Read the model definition and answer for the solid it produces. Units are mm, in the model's axes. A direction names the side the tool comes from. Give positions to 0.01 mm unless a question says otherwise; leave off trailing zeros. Write each loop counter-clockwise with the first axis right and the second up, starting at its lowest first coordinate (ties: lowest second). Pieces come first, ordered by that corner, then holes. Notation, with made-up numbers: M -23,35 L 12,35 A21 ccw 12,65 Z; hole C 2,28.25 d11. An arc over 180 degrees is marked long. Put each result on its own line as item: value.
from build123d import *

# Parameters (mm, degrees)
ESBO_O1_R                                            = 7
RESSALTO_EXTRUS_O1_DEPTH                             = 7.9375
ESCAREADO_PARA_PARAFUSO_DE_M_QUINA_COM_C_D           = 5.5
ESCAREADO_PARA_PARAFUSO_DE_M_QUINA_COM_C_DEPTH       = 30
ESCAREADO_PARA_PARAFUSO_DE_M_QUINA_COM_C_CSINK_D     = 10.4
ESCAREADO_PARA_PARAFUSO_DE_M_QUINA_COM_C_CSINK_ANGLE = 90
ESCAREADO_PARA_PARAFUSO_DE_M_QUINA_COM_C_TIP         = 1.652366702
ESCAREADO_PARA_PARAFUSO_DE_M_QUINA_C_2_D             = 6.6
ESCAREADO_PARA_PARAFUSO_DE_M_QUINA_C_2_DEPTH         = 30
ESCAREADO_PARA_PARAFUSO_DE_M_QUINA_C_2_CSINK_D       = 12.6
ESCAREADO_PARA_PARAFUSO_DE_M_QUINA_C_2_CSINK_ANGLE   = 90
ESCAREADO_PARA_PARAFUSO_DE_M_QUINA_C_2_TIP           = 1.982840043
BROCA_DE_ROSQUEAR_PARA_TARRAXA_DE_M5X0_8_D           = 4.2
BROCA_DE_ROSQUEAR_PARA_TARRAXA_DE_M5X0_8_DEPTH       = 20
BROCA_DE_ROSQUEAR_PARA_TARRAXA_DE_M5X0_8_TIP         = 1.2618073
BROCA_DE_ROSQUEAR_PARA_TARRAXA_DE_M5_2_D             = 4.2
BROCA_DE_ROSQUEAR_PARA_TARRAXA_DE_M5_2_DEPTH         = 20
BROCA_DE_ROSQUEAR_PARA_TARRAXA_DE_M5_2_TIP           = 1.2618073
BROCA_DE_ROSQUEAR_PARA_TARRAXA_DE_M6X1_0_D           = 5
BROCA_DE_ROSQUEAR_PARA_TARRAXA_DE_M6X1_0_DEPTH       = 15
BROCA_DE_ROSQUEAR_PARA_TARRAXA_DE_M6X1_0_TIP         = 1.502151548
FILLET1_R                                            = 6
SKETCH7_R                                            = 9.5
CUT_EXTRUDE4_DEPTH                                   = 5


with BuildPart() as part:
    # Esboço1 → Ressalto-extrusão1 (new, symmetric)
    with BuildSketch(Plane(origin=(0, 0, 0), x_dir=(0, 0, -1), z_dir=(1, 0, 0))):
        Polygon((-10, 38.5), (-40, 38.5), (-40, 23.5), (-40, 17.44427191), (-32, 8.5), (-32, -16.5), (73, -16.5), (73, 27.5), (-10, 27.5), align=None)
        with Locations((-25, 23.5)):
            Circle(ESBO_O1_R, mode=Mode.SUBTRACT)
    extrude(amount=RESSALTO_EXTRUS_O1_DEPTH, both=True)

    # Escareado para parafuso de m_quina com c
    with Locations(Plane(origin=(33.0625, -10.251665499, 40.070399895), x_dir=(1, 0, 0), z_dir=(0, 0, 1))):
        with Locations((-33.0625, 13.751665499), (-33.0625, -1.248334501), (33.0625, -1.248334501), (33.0625, 13.751665499)):
            CounterSinkHole(ESCAREADO_PARA_PARAFUSO_DE_M_QUINA_COM_C_D / 2, ESCAREADO_PARA_PARAFUSO_DE_M_QUINA_COM_C_CSINK_D / 2, depth=ESCAREADO_PARA_PARAFUSO_DE_M_QUINA_COM_C_DEPTH, counter_sink_angle=ESCAREADO_PARA_PARAFUSO_DE_M_QUINA_COM_C_CSINK_ANGLE)
            with Locations((0, 0, -(ESCAREADO_PARA_PARAFUSO_DE_M_QUINA_COM_C_DEPTH + ESCAREADO_PARA_PARAFUSO_DE_M_QUINA_COM_C_TIP / 2))):  # 118° drill point
                Cone(0, ESCAREADO_PARA_PARAFUSO_DE_M_QUINA_COM_C_D / 2, ESCAREADO_PARA_PARAFUSO_DE_M_QUINA_COM_C_TIP, mode=Mode.SUBTRACT)

    # Escareado para parafuso de m_quina c 2
    with Locations(Plane(origin=(33.0625, -23.5, -11.460196829), x_dir=(-1, 0, 0), z_dir=(0, -1, 0))):
        with Locations((33.06, 53.539803171), (33.06, -3.413475694), (-33.06, -3.413475694), (-33.06, 49.586524306)):
            CounterSinkHole(ESCAREADO_PARA_PARAFUSO_DE_M_QUINA_C_2_D / 2, ESCAREADO_PARA_PARAFUSO_DE_M_QUINA_C_2_CSINK_D / 2, depth=ESCAREADO_PARA_PARAFUSO_DE_M_QUINA_C_2_DEPTH, counter_sink_angle=ESCAREADO_PARA_PARAFUSO_DE_M_QUINA_C_2_CSINK_ANGLE)
            with Locations((0, 0, -(ESCAREADO_PARA_PARAFUSO_DE_M_QUINA_C_2_DEPTH + ESCAREADO_PARA_PARAFUSO_DE_M_QUINA_C_2_TIP / 2))):  # 118° drill point
                Cone(0, ESCAREADO_PARA_PARAFUSO_DE_M_QUINA_C_2_D / 2, ESCAREADO_PARA_PARAFUSO_DE_M_QUINA_C_2_TIP, mode=Mode.SUBTRACT)

    # Broca de rosquear para tarraxa de M5x0.8
    with Locations(Plane(origin=(33.0625, 48.5, -11.460196829), x_dir=(1, 0, 0), z_dir=(0, 1, 0))):
        with Locations((33.06, -45.460196829), (-33.065, -45.460196829)):
            Hole(BROCA_DE_ROSQUEAR_PARA_TARRAXA_DE_M5X0_8_D / 2, depth=BROCA_DE_ROSQUEAR_PARA_TARRAXA_DE_M5X0_8_DEPTH)
            with Locations((0, 0, -(BROCA_DE_ROSQUEAR_PARA_TARRAXA_DE_M5X0_8_DEPTH + BROCA_DE_ROSQUEAR_PARA_TARRAXA_DE_M5X0_8_TIP / 2))):  # 118° drill point
                Cone(0, BROCA_DE_ROSQUEAR_PARA_TARRAXA_DE_M5X0_8_D / 2, BROCA_DE_ROSQUEAR_PARA_TARRAXA_DE_M5X0_8_TIP, mode=Mode.SUBTRACT)

    # Broca de rosquear para tarraxa de M5 2
    with Locations(Plane(origin=(33.0625, -10.251665499, 0), x_dir=(-1, 0, 0), z_dir=(0, 0, -1))):
        with Locations((-33.06, 43.751665499), (33.065, 43.751665499)):
            Hole(BROCA_DE_ROSQUEAR_PARA_TARRAXA_DE_M5_2_D / 2, depth=BROCA_DE_ROSQUEAR_PARA_TARRAXA_DE_M5_2_DEPTH)
            with Locations((0, 0, -(BROCA_DE_ROSQUEAR_PARA_TARRAXA_DE_M5_2_DEPTH + BROCA_DE_ROSQUEAR_PARA_TARRAXA_DE_M5_2_TIP / 2))):  # 118° drill point
                Cone(0, BROCA_DE_ROSQUEAR_PARA_TARRAXA_DE_M5_2_D / 2, BROCA_DE_ROSQUEAR_PARA_TARRAXA_DE_M5_2_TIP, mode=Mode.SUBTRACT)

    # Broca de rosquear para tarraxa de M6x1.01
    with Locations(Plane(origin=(33.0625, 27.5, -11.460196829), x_dir=(1, 0, 0), z_dir=(0, 1, 0))):
        with Locations((33.06, 49.539803171), (-33.06, 53.539803171), (-33.06, -3.413475694), (33.06, -3.413475694)):
            Hole(BROCA_DE_ROSQUEAR_PARA_TARRAXA_DE_M6X1_0_D / 2, depth=BROCA_DE_ROSQUEAR_PARA_TARRAXA_DE_M6X1_0_DEPTH)
            with Locations((0, 0, -(BROCA_DE_ROSQUEAR_PARA_TARRAXA_DE_M6X1_0_DEPTH + BROCA_DE_ROSQUEAR_PARA_TARRAXA_DE_M6X1_0_TIP / 2))):  # 118° drill point
                Cone(0, BROCA_DE_ROSQUEAR_PARA_TARRAXA_DE_M6X1_0_D / 2, BROCA_DE_ROSQUEAR_PARA_TARRAXA_DE_M6X1_0_TIP, mode=Mode.SUBTRACT)

    # Fillet1
    # the kernel refuses this fillet: 6 mm, written as the material it adds along each edge
    with BuildSketch(Plane(origin=(7.9375, 27.5, 10), x_dir=(0, 1, 0), z_dir=(-1, 0, 0))) as fillet1_piece_1_section:
        with BuildLine():
            CenterArc((FILLET1_R, FILLET1_R), FILLET1_R, 180, 90)
            Line((0, FILLET1_R), (0, 0))
            Line((0, 0), (FILLET1_R, 0))
        make_face()
    fillet1_piece_1 = extrude(amount=15.875, mode=Mode.PRIVATE)
    fillet1_piece_1 = fillet1_piece_1 - Plane(origin=(-0.0025, 33.5, 8.627789353), x_dir=(1, 0, 0), z_dir=(0, 0, 1)) * Cylinder(2.1, 56, mode=Mode.PRIVATE)
    add(fillet1_piece_1)

    # Sketch7 → Cut-Extrude4 (cut)
    with BuildSketch(Plane(origin=(7.9375, 0, 0), x_dir=(0, 0, -1), z_dir=(1, 0, 0))):
        with Locations((39.5, 5.5)):
            Circle(SKETCH7_R)
    extrude(amount=-CUT_EXTRUDE4_DEPTH, mode=Mode.SUBTRACT)


solid = part.part
(1) Section A-A on y = 23.5 is taken. Determine the outline of the cut face in (x, z), and give its area (3 significant figures).
Result:
outline: M -7.94,-73 L 7.94,-73 L 7.94,18 L -7.94,18 Z; M -7.94,32 L 7.94,32 L 7.94,40 L -7.94,40 Z; hole C 0,-65 d5; hole C 0,-8.05 d5
area: 1,530 mm²
(2) Section D-D on y = -6.5 is taken. Determine the outline of the cut face in (x, z), and give its area (3 significant figures).
Result:
outline: M -7.94,-73 L 7.94,-73 L 7.94,32 L -7.94,32 Z; hole C 0,-65 d6.6; hole C 0,-8.05 d6.6
area: 1,600 mm²
(3) Given pin 1 Ø9.5 at (y, z) = (5, -44) entering from +X; pin 2 Ø2.5 at (x, y) = (-2, 35) entering from -Z; pin 3 Ø10 at (y, z) = (33, -47) entering from -X; pin 4 Ø6 at (x, z) = (0, -8.05) entering from -Y, each flat-ended and moving along its own axis, determine where each tip first touches the part or whether it passes through.
Result:
pin 1: stops at x = 2.94
pin 2: stops at z = 10
pin 3: passes through
pin 4: stops at y = 6.68
(4) Which of the six approach directions +Z, -Z, +X, -X, +Y, -Y give full straight-line access (tool end or side, diameter ignored) to faces 1 (the face through (0.45, 33.43, 36.05)), 2 (the face through (5.472, 8.354, -48.561)), 3 (the face through (0, 36, 10))?
Result:
face 1: +Y
face 2: +X
face 3: -Z, +X, -X, +Y
(5) Section B-B on x = 6.25 is taken. Determine the outline of the cut face in (y, z), and give its area (3 significant figures).
Result:
outline: M -16.5,-73 L 27.5,-73 L 27.5,4 A6 cw 33.5,10 L 38.5,10 L 38.5,40 L 17.44,40 L 8.5,32 L -16.5,32 Z; hole C 5.5,-39.5 d19; hole C 23.5,25 d14
area: 4,640 mm²
(6) Section C-C on z = -39.5 is taken. Determine the outline of the cut face in (x, y).
Result:
outline: M -7.94,-16.5 L 7.94,-16.5 L 7.94,-4 L 2.94,-4 L 2.94,15 L 7.94,15 L 7.94,27.5 L -7.94,27.5 Z
(7) For a pull along Y with two mould halves and no side action, classify faces 4 (the face through (-0.062, 3.974, 8.705)), 5 (the face through (0, 11, -65)), 6 (the face through (0.111, 13.035, 36.056)) as +Y half, -Y half, draft (parallel to the pull), parting line (faces both ways), or undercut.
Result:
face 4: undercut
face 5: +Y half
face 6: -Y half
(8) Straight lines are drawn through the part: line 1 along Y through (x, z) = (0, 24.5); line 2 along Y through (x, z) = (0, 15); line 3 along X through (y, z) = (33.5, 13.25). For each, find the intervals that lie inside material, in ascending order. Write a range as from..to.
Result:
line 1: y = -16.5..-14.25, -8.75..0.75, 6.25..16.52, 30.48..38.5
line 2: y = -16.5..-14.25, -8.75..0.75, 6.25..31.4, 35.6..38.5
line 3: x = -7.94..-2.1, 2.1..7.94
